Study the drawing (mm; zero at the part's minimum x, y, z) and answer. Round coordinates to 2 decimals unless told otherwise and drop trailing zeros. Order: outer loops, then holes, each group sorted by start corner. A loop starts at its lowest first (then second) coordinate and runs counter-clockwise, first axis right, second up. Notation, with made-up numbers: (-6.75, 18) - (37.25, 18) arc R31 ccw to (37.25, 50) - close; hole circle Ø5 at (80, 67.5). An arc over 180 degrees is marked (long way). Put each result on its own line as item: value. Start each with the question number.
Q1. Section B-B on y = 19.25 is taken. Give the vertices of the cut face in (x, z).
Q2. Section C-C on z = 100.5 is taken. Give the vertices of the cut face in (x, y) (1 decimal).
Q3. Section A-A on x = 18.5 is taken. Give the vertices of the cut face in (y, z) (1 decimal).
Q4. This flat-tipped pin is pushed along its axis until it touches: pin 1 Ø3.5 at (x, z) = (12.7, 38.1) entering from +Y. Where does it stop, or does it pass through?
Q5. For a pull along X with two mould halves and no side action, classify the marked faces 1, 2, 3 and 4 as pulls with the +X half, pulls with the -X half, needs draft (parallel to the pull), parting line crosses it, or undercut.
Q6. Find the intervals of material crossed by line 1 along X through (y, z) = (20.25, 159); line 2 along Y through (x, z) = (1.75, 96.5) (1 decimal); line 3 along X through (y, z) = (1.35, 139.7), in increasing order. Write a range as from..to.
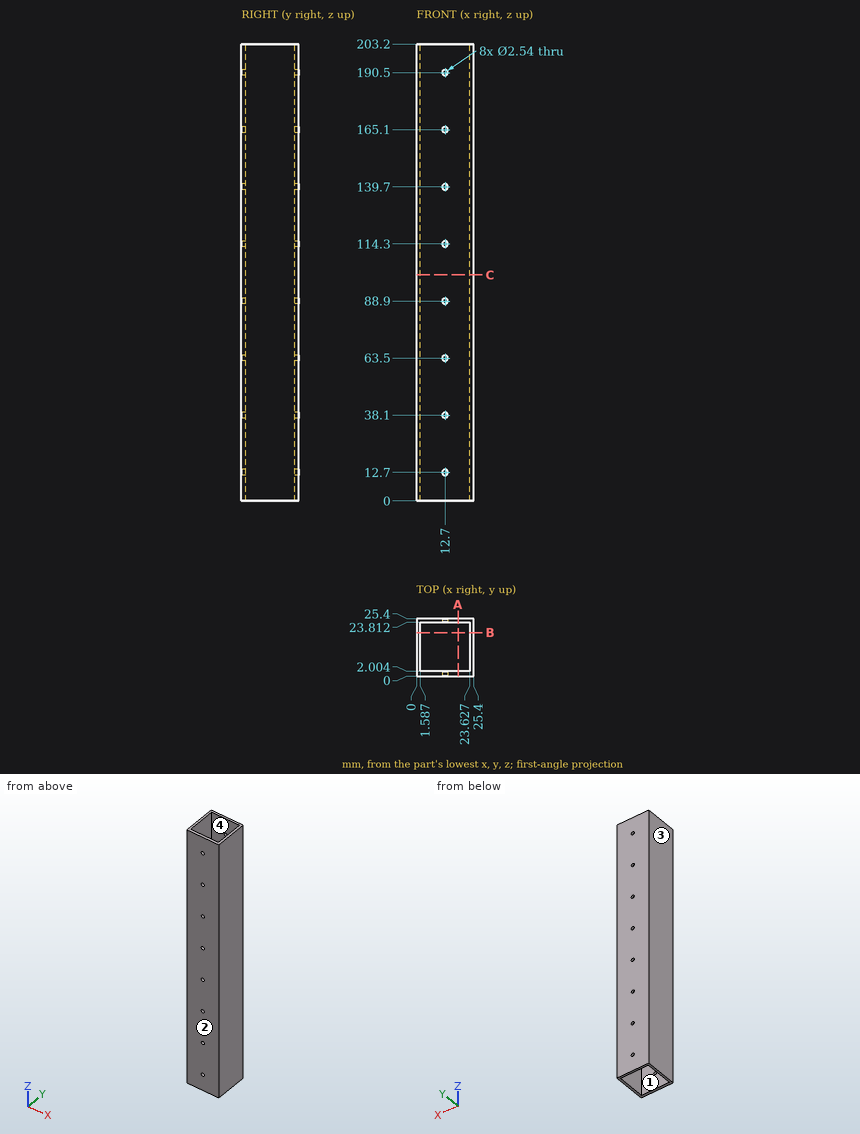
Findings:
1. outline: (0, 0) - (1.59, 0) - (1.59, 203.2) - (0, 203.2) - close; (23.63, 0) - (25.4, 0) - (25.4, 203.2) - (23.63, 203.2) - close
2. outline: (0, 0) - (25.4, 0) - (25.4, 25.4) - (0, 25.4) - close; hole (1.6, 2) - (23.6, 2) - (23.6, 23.8) - (1.6, 23.8) - close
3. outline: (0, 0) - (2, 0) - (2, 203.2) - (0, 203.2) - close; (23.8, 0) - (25.4, 0) - (25.4, 203.2) - (23.8, 203.2) - close
4. pin 1: y = 25.4
5. face 1: undercut
5. face 2: needs draft
5. face 3: pulls with the -X half
5. face 4: undercut
6. line 1: 0..1.59, 23.63..25.4
6. line 2: 0..2, 23.8..25.4
6. line 3: 0..11.43, 13.97..25.4
